Part print with two shaded views. Sizes in mm from the minimum x, y, z corner. Give positions to 0.01 mm unless a question says otherwise; leave off trailing zeros. Write each loop counter-clockwise with the first axis right and the second up, starting at its lowest first coordinate (ties: lowest second). Pieces come first, ordered by that corner, then holes. Notation, with made-up numbers: M 49.5,34 L 74.5,34 A12 ccw 74.5,45 Z; hole C -23.75,-35 d2. An arc over 180 degrees is marked long. Return JSON: item names as keys, results as strings. Group by question number.
Q1. Flat gauge pins, fed straight in: pin 1 Ø1.5 at (y, z) = (3, 10.5) entering from +X; pin 2 Ø0.7 at (x, y) = (1, 3) entering from -Z; pin 3 Ø0.7 at (x, z) = (2.5, 6.5) entering from +Y. Where does each tip first touch, or does it go through?
Q2. Band-saw the part on B-B, the plane z = 9.6. Give the cut face in (x, y).
Q3. Wall check: probe 1 along Z at (x, y) = (1.25, 3.1); probe 2 along Z at (x, y) = (5.75, 0.95); probe 3 along X at (y, z) = (5.3, 2). Give the ranges that are in metal, low to high.
Q4. Band-saw the part on A-A, the plane x = 3. Give the cut face in (y, z).
Q5. Band-saw the part on D-D, the plane x = 5.1. Give the cut face in (y, z), then the cut area to 3 significant figures.
Q6. Pull direction Z, two halves, no side cores. Call the marked faces 1, 2 and 3: +Z half, -Z half, draft (parallel to the pull), parting line (faces both ways), or undercut.
Q7. Band-saw the part on C-C, the plane y = 3.3. Give the cut face in (x, z) (3 decimals).
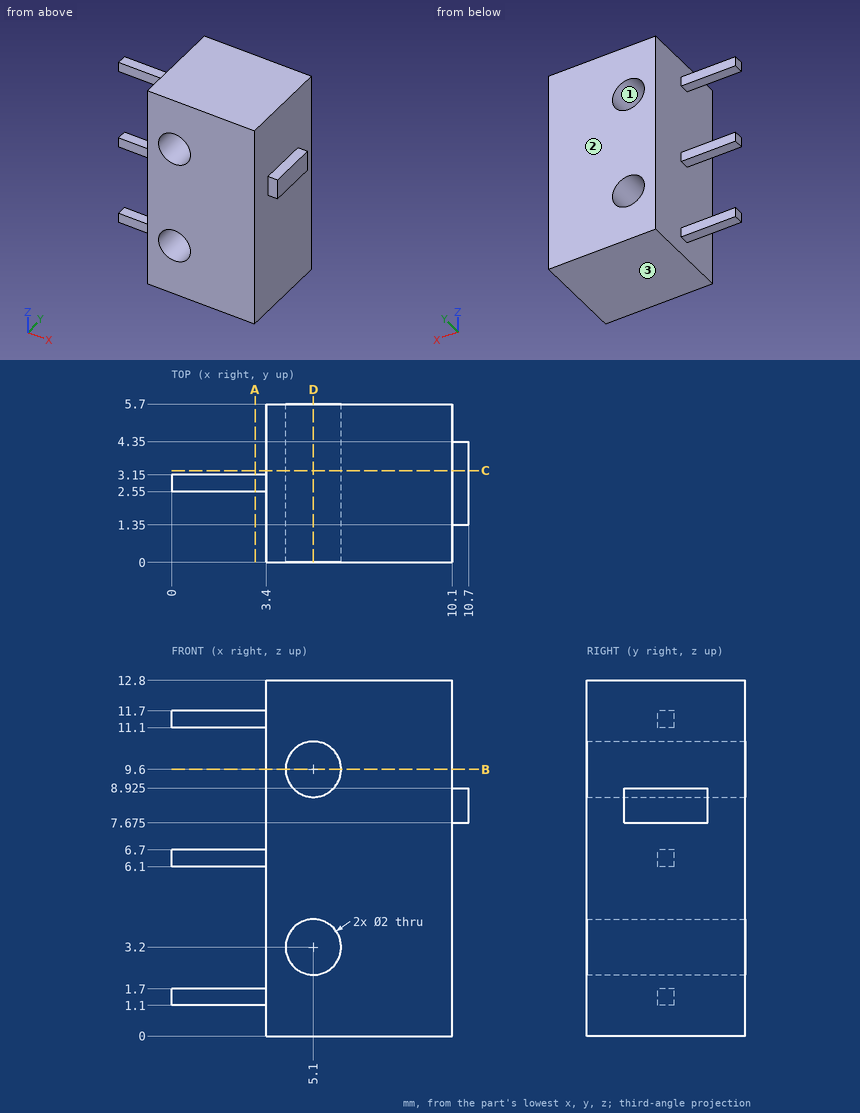
From the geometry:
{
 "1": {"pin 1": "stops at x = 10.1", "pin 2": "stops at z = 1.1", "pin 3": "stops at y = 3.15"},
 "2": {"outline": "M 3.4,0 L 4.1,0 L 4.1,5.7 L 3.4,5.7 Z; M 6.1,0 L 10.1,0 L 10.1,5.7 L 6.1,5.7 Z"},
 "3": {"probe 1": "z = 1.1 to 1.7, 6.1 to 6.7, 11.1 to 11.7", "probe 2": "z = 0 to 2.44, 3.96 to 8.84, 10.36 to 12.8", "probe 3": "x = 3.4 to 10.1"},
 "4": {"outline": "M 2.55,1.1 L 3.15,1.1 L 3.15,1.7 L 2.55,1.7 Z; M 2.55,6.1 L 3.15,6.1 L 3.15,6.7 L 2.55,6.7 Z; M 2.55,11.1 L 3.15,11.1 L 3.15,11.7 L 2.55,11.7 Z"},
 "5": {"outline": "M 0,0 L 5.7,0 L 5.7,2.2 L 0,2.2 Z; M 0,4.2 L 5.7,4.2 L 5.7,8.6 L 0,8.6 Z; M 0,10.6 L 5.7,10.6 L 5.7,12.8 L 0,12.8 Z", "area": "50.2 mm^2"},
 "6": {"face 1": "undercut", "face 2": "draft", "face 3": "-Z half"},
 "7": {"outline": "M 3.4,0 L 10.1,0 L 10.1,7.675 L 10.7,7.675 L 10.7,8.925 L 10.1,8.925 L 10.1,12.8 L 3.4,12.8 Z; hole C 5.1,3.2 d2; hole C 5.1,9.6 d2"}
}
